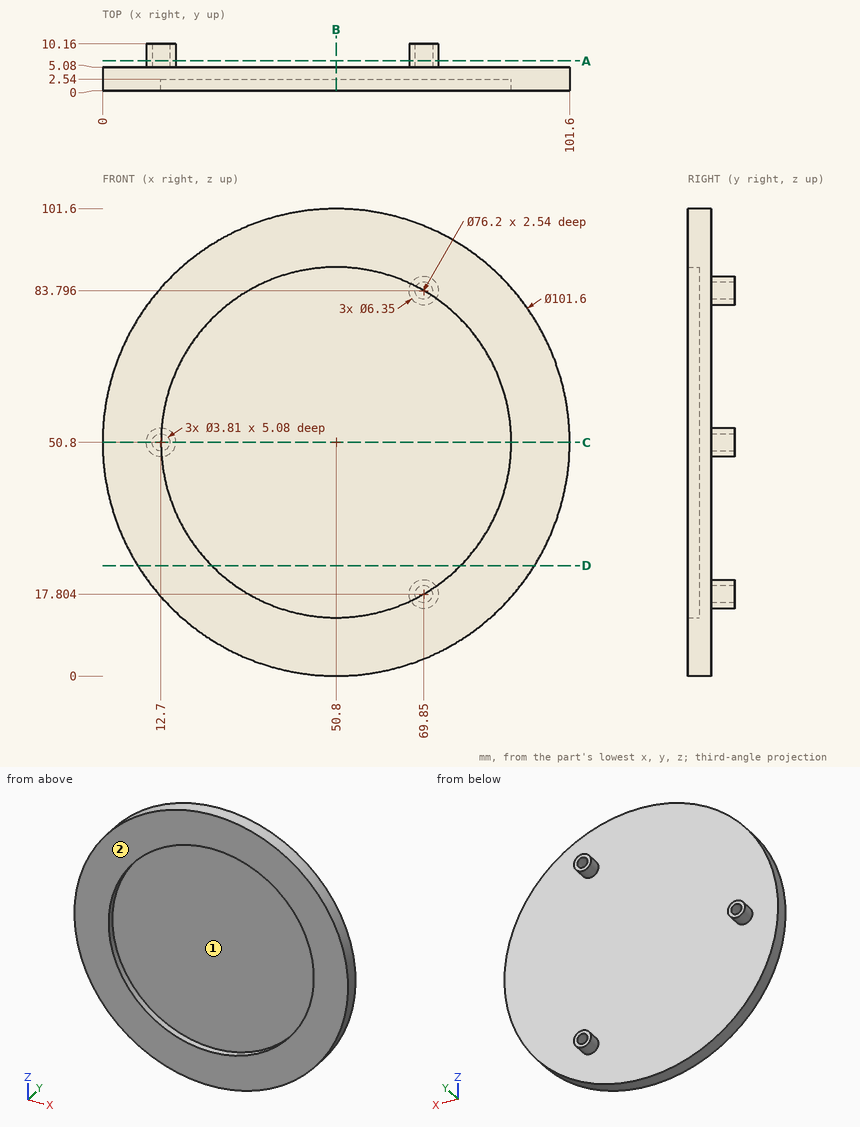
Geometry check sheet. Reference: drawing and pictorial views, mm from the part's lowest x, y, z. Round coordinates to 2 decimals unless told otherwise and drop trailing zeros. Write each loop counter-clockwise with the first axis right and the second up, starting at its lowest first coordinate (ties: lowest second). Pieces come first, ordered by that corner, then holes.
Item 1: Material ranges on line 1 along Z through (x, y) = (71, 8) (1 decimal); line 2 along Y through (x, z) = (15.5, 66); line 3 along Y through (x, z) = (19, 56), recorded low to high.
Determined:
line 1: z = 14.8 to 16.3, 19.3 to 20.8, 80.8 to 82.3, 85.3 to 86.8
line 2: y = 0 to 5.08
line 3: y = 2.54 to 5.08
Item 2: Section check C-C (z = 50.8). Record the boundary of the cut face in (x, y) (1 decimal).
Determined:
outline: (0, 0) - (12.7, 0) - (12.7, 2.5) - (88.9, 2.5) - (88.9, 0) - (101.6, 0) - (101.6, 5.1) - (15.9, 5.1) - (15.9, 10.2) - (14.6, 10.2) - (14.6, 5.1) - (10.8, 5.1) - (10.8, 10.2) - (9.5, 10.2) - (9.5, 5.1) - (0, 5.1) - close
Item 3: Mould release check, pull along X, two halves, no side actions. Record for the marked faces 1 and 2: +X half, -X half, draft (parallel to the pull), parting line (faces both ways), or undercut.
Determined:
face 1: undercut
face 2: draft
Item 4: Go/stop test with flat-tipped pins: pin 1 Ø6 at (x, z) = (69.85, 17.8) entering from -Y; pin 2 Ø4 at (x, y) = (43, 7) entering from -Z; pin 3 Ø1.5 at (x, y) = (63, 2) entering from +Z; pin 4 Ø4 at (x, z) = (86.5, 83) entering from +Y. Record where each tip stops, or that it passes through.
Determined:
pin 1: stops at y = 0
pin 2: stops at z = 0.52
pin 3: stops at z = 100.29
pin 4: stops at y = 5.08
Item 5: Section check D-D (z = 24). Record the boundary of the cut face in (x, y) (1 decimal).
Determined:
outline: (7.6, 0) - (23.7, 0) - (23.7, 2.5) - (77.9, 2.5) - (77.9, 0) - (94, 0) - (94, 5.1) - (7.6, 5.1) - close
Item 6: Section check A-A (y = 6.5). Give the number of separate pieces and of enclosed holes in the cut face.
Determined:
separate pieces: 3
enclosed holes: 3
Item 7: Section check B-B (x = 50.8). Record the boundary of the cut face in (y, z).
Determined:
outline: (0, 0) - (5.08, 0) - (5.08, 101.6) - (0, 101.6) - (0, 88.9) - (2.54, 88.9) - (2.54, 12.7) - (0, 12.7) - close
